Model file for the job. Use its own axes, mm. A direction names the side the tool comes from. Round coordinates to 2 decimals unless told otherwise and drop trailing zeros. Order: outer loops, then holes, each group sorted by start corner. A loop starts at its lowest first (then second) coordinate and runs counter-clockwise, first axis right, second up. Notation, with made-up numbers: (20, 71.25) -> (76, 71.25) arc R26 ccw to (76, 107.25) -> close; hole circle Ø9 at (-35.5, -31). An arc over 180 degrees is marked (long way). Put each result on its own line as item: value. Start each with the question number.
Q1. Cut at C-C, the plane x = -8. List the corners of the cut face in (y, z).
Q2. Probe L1, parallel to Y at x = 6, z = 31.5; L2, parallel to Y at x = 2, z = -7; L3, parallel to X at y = 36, z = -8. List the from-to ranges inside material, lowest first.
Q3. Pull direction Y, two halves, no side cores. Call faces 1 (the face through (5, 4, 33)), 2 (the face through (4.93, 46.536, -6.825)), 3 (the face through (5, 51, 34)), 4 (the face through (-9, 28, 25)): released by +Y, released by -Y, zero draft, split by the parting line, or undercut.
Q4. Flat gauge pins, fed straight in: P1, Ø1.5, axis at y = 0, z = 14, coming from the +X side; P2, Ø7.5, axis at y = 39.5, z = -6, coming from the -X side; P3, Ø1.5, axis at y = 33.5, z = 28.5, coming from the -X side; P4, Ø2.5, axis at y = 48, z = 31.5, coming from the -X side. Where does each tip first touch, or does it go through?
Q5. Cut at B-B, the plane z = 31.5. List the corners of the cut face in (x, y), and give its area (3 significant figures).
Q6. Cut at A-A, the plane x = 1. List the corners of the cut face in (y, z).
Q7. 3-axis set-ups, long thin cutter, end or side, ignore diameter. For faces 5 (the face through (10, 28, 13)), 6 (the face through (0, 28, 32)), 7 (the face through (0, 1, 12)), 8 (the face through (-18.6, 29, 12)), 9 (the face through (0, 56, 12)): which of +Z, -Z, +X, -X, +Y, -Y reach the whole face in a straight line?
Q8. Cut at D-D, the plane y = 27. List the corners of the cut face in (x, z), and give its area (3 significant figures).
from build123d import *

# Parameters (mm, degrees)
BOSS_EXTRUDE1_DEPTH = 25
SKETCH2_W           = 18.6
SKETCH2_H           = 25
BOSS_EXTRUDE2_DEPTH = 2
FILLET1_R           = 0.5
SKETCH3_W           = 12.5
SKETCH3_H           = 50
SKETCH3_W_2         = 10
BOSS_EXTRUDE3_DEPTH = 10
FILLET2_R           = 3
SKETCH4_R           = 1.5
CUT_EXTRUDE1_DEPTH  = 71.249270459
FILLET3_R           = 5


with BuildPart() as part:
    # Sketch1 → Boss-Extrude1 (new body)
    with BuildSketch(Plane.XY):
        with BuildLine():
            Line((-18.6, 0), (0, 0))
            Line((0, 0), (0, 58))
            Line((0, 58), (-18.6, 58))
            Line((-18.6, 58), (-18.6, 54.737646833))
            ThreePointArc((-18.6, 54.737646833), (-7.823111162, 52.413626985), (-3, 42.5))
            ThreePointArc((-3, 42.5), (-7.823111162, 32.586373015), (-18.6, 30.262353167))
            Line((-18.6, 30.262353167), (-18.6, 27.737646833))
            ThreePointArc((-18.6, 27.737646833), (-7.823111162, 25.413626985), (-3, 15.5))
            ThreePointArc((-3, 15.5), (-7.823111162, 5.586373015), (-18.6, 3.262353167))
            Line((-18.6, 3.262353167), (-18.6, 0))
        make_face()
    extrude(amount=BOSS_EXTRUDE1_DEPTH)

    # Sketch2 → Boss-Extrude2 (add)
    with BuildSketch(Plane.XZ):
        with Locations((-9.3, 12.5)):
            Rectangle(SKETCH2_W, SKETCH2_H)
    extrude(amount=BOSS_EXTRUDE2_DEPTH)

    # Fillet1
    fillet1_edges = [part.edges().sort_by_distance(p)[0] for p in [
        (-18.6, 3.262353167, 12.5),
        (-18.6, 27.737646833, 12.5),
        (-18.6, 30.262353167, 12.5),
        (-18.6, 54.737646833, 12.5),
    ]]
    fillet(fillet1_edges, radius=FILLET1_R)

    # Sketch3 → Boss-Extrude3 (add)
    with BuildSketch(Plane(origin=(0, 0, 0), x_dir=(0, 0, -1), z_dir=(1, 0, 0))):
        with Locations((-18.75, 28)):
            Rectangle(SKETCH3_W, SKETCH3_H)
        with Locations((-6.25, 28)):
            Rectangle(SKETCH3_W, SKETCH3_H)
        with Locations((5, 28)):
            Rectangle(SKETCH3_W_2, SKETCH3_H)
        with Locations((-30, 28)):
            Rectangle(SKETCH3_W_2, SKETCH3_H)
    extrude(amount=BOSS_EXTRUDE3_DEPTH)

    # Fillet2
    fillet2_edges = [part.edges().sort_by_distance(p)[0] for p in [
        (0, 28, 0),
        (0, 28, 25),
    ]]
    fillet(fillet2_edges, radius=FILLET2_R - 0.0001)  # a hair under: the kernel refuses the full size

    # Sketch4 → Cut-Extrude1 (cut, through all)
    with BuildSketch(Plane.ZY):
        with Locations((-6.5, 48)):
            Circle(SKETCH4_R)
        with Locations((-6.5, 8)):
            Circle(SKETCH4_R)
        with Locations(Location((31.5, 8, 0), (0, 0, 180))):
            Circle(SKETCH4_R)
        with Locations(Location((31.5, 48, 0), (0, 0, 180))):
            Circle(SKETCH4_R)
    extrude(amount=-CUT_EXTRUDE1_DEPTH, mode=Mode.SUBTRACT)

    # Fillet3
    fillet3_edges = [part.edges().sort_by_distance(p)[0] for p in [
        (5, 3, 35),
        (5, 3, -10),
        (5, 53, -10),
        (5, 53, 35),
    ]]
    fillet(fillet3_edges, radius=FILLET3_R)


solid = part.part
Ans:
1. outline: (-2, 0) -> (5.45, 0) -> (5.45, 25) -> (-2, 25) -> close; (25.55, 0) -> (32.45, 0) -> (32.45, 25) -> (25.55, 25) -> close; (52.55, 0) -> (58, 0) -> (58, 25) -> (52.55, 25) -> close
2. L1: y = 3.23 to 6.5, 9.5 to 46.5, 49.5 to 52.77
2. L2: y = 3.42 to 6.59, 9.41 to 46.59, 49.41 to 52.58
2. L3: x = 0 to 10
3. face 1: released by -Y
3. face 2: undercut
3. face 3: released by +Y
3. face 4: zero draft
4. P1: stops at x = 0
4. P2: stops at x = -0.1
4. P3: stops at x = -0.01
4. P4: passes through
5. outline: (0, 3.23) -> (10, 3.23) -> (10, 6.5) -> (0, 6.5) -> close; (0, 9.5) -> (10, 9.5) -> (10, 46.5) -> (0, 46.5) -> close; (0, 49.5) -> (10, 49.5) -> (10, 52.77) -> (0, 52.77) -> close
5. area: 435 mm^2
6. outline: (3, -5) arc R5 ccw to (8, -10) -> (48, -10) arc R5 ccw to (53, -5) -> (53, 30) arc R5 ccw to (48, 35) -> (8, 35) arc R5 ccw to (3, 30) -> close; hole circle Ø3 at (8, -6.5); hole circle Ø3 at (8, 31.5); hole circle Ø3 at (48, -6.5); hole circle Ø3 at (48, 31.5)
7. face 5: +Z, -Z, +X, +Y, -Y
7. face 6: +Z, -X, +Y, -Y
7. face 7: +Z, -Z, +X, -Y
7. face 8: +Z, -Z, -X, +Y, -Y
7. face 9: +Z, -Z, +X, +Y
8. outline: (-10.45, 0) -> (-3, 0) arc R3 cw to (0, -3) -> (0, -10) -> (10, -10) -> (10, 35) -> (0, 35) -> (0, 28) arc R3 cw to (-3, 25) -> (-10.45, 25) -> close
8. area: 715 mm^2
